Check sheet for the modelled part. Datum: model origin and axes. Units: mm. A direction names the side the tool comes from. Give positions to 0.01 mm unless a question says otherwise; leave off trailing zeros. Order: outer loops, then holes, each group sorted by start corner. A loop starts at its lowest first (then second) coordinate and runs counter-clockwise, first axis right, second up.
Item 1: Sectioned sample at D-D on z = 2.5. Count the separate pieces of the cut face and the enclosed holes in it, and give its area (3 significant figures).
Item 2: Release check for a two-part mould opening along X. For faces 5 (the flat face through (51.3, 6, 7)), 6 (the flat face through (5, 39.1, 5)), 7 (the flat face through (8.7, 18, 7)) record: released by +X, released by -X, zero draft, split by the parting line, or undercut.
Item 3: Sectioned sample at C-C on x = 4.5. Record the boundary of the cut face in (y, z).
Item 4: Access from +Z, -Z, +X, -X, +Y, -Y to the whole of each face (thin tool, end or side, straight path). Record for faces 1 (the flat face through (7, 26.4, 5)), 2 (the flat face through (47, 49.9, 7)), 3 (the flat face through (50, 25, 1)), 4 (the flat face through (47, 39.9, 7)).
Item 5: Gauge pin test, flat ends, axial feed: P1, Ø4.5, axis at x = 4, z = 9, coming from the +Y side; P2, Ø12, axis at x = 39, y = 31.5, coming from the +Z side; P3, Ø2, axis at x = 5, z = 6, coming from the -Y side. Record the tip position at first contact, or that the pin passes through.
Item 6: Material ranges on line 1 along Y through (x, z) = (4.5, 8.75); line 2 along Y through (x, z) = (2, 4.5); line 3 along X through (y, z) = (40, 7.75), recorded low to high.
Item 7: Sectioned sample at A-A on z = 10.5. Record the boundary of the cut face in (x, y).
Item 8: Sectioned sample at B-B on y = 4.5. Record the boundary of the cut face in (x, z), and give its area (3 significant figures).
from build123d import *

# Parameters (mm, degrees)
CROQUIS1_W              = 50
CROQUIS1_H              = 50
SALIENTE_EXTRUIR1_DEPTH = 1.2
CROQUIS2_W              = 9
CROQUIS2_H              = 10
SALIENTE_EXTRUIR2_DEPTH = 11.8
CROQUIS3_W              = 27.94
CROQUIS3_H              = 2.54
CROQUIS3_W_2            = 2.54
CROQUIS3_H_2            = 15.24
CROQUIS3_H_3            = 10.16
CROQUIS3_W_3            = 5.08
SALIENTE_EXTRUIR3_DEPTH = 8


with BuildPart() as part:
    # Croquis1 → Saliente-Extruir1 (new body)
    with BuildSketch(Plane.XY):
        with Locations((25, 25)):
            Rectangle(CROQUIS1_W, CROQUIS1_H)
    extrude(amount=SALIENTE_EXTRUIR1_DEPTH)

    # Croquis2 → Saliente-Extruir2 (add)
    with BuildSketch(Plane.XY.offset(1.2)):
        with Locations((46.8, 5.8)):
            Rectangle(CROQUIS2_W, CROQUIS2_H)
        with Locations((46.8, 18.4)):
            Rectangle(CROQUIS2_W, CROQUIS2_H)
        with Locations((46.8, 44.9)):
            Rectangle(CROQUIS2_W, CROQUIS2_H)
        with Locations((4.2, 44.9)):
            Rectangle(CROQUIS2_W, CROQUIS2_H)
        with Locations((4.2, 18.1)):
            Rectangle(CROQUIS2_W, CROQUIS2_H)
    extrude(amount=SALIENTE_EXTRUIR2_DEPTH)

    # Croquis3 → Saliente-Extruir3 (add)
    with BuildSketch(Plane.XY.offset(1.2)):
        with Locations((14.57, 2.07)):
            Rectangle(CROQUIS3_W, CROQUIS3_H)
        with Locations((4.57, 31.48)):
            Rectangle(CROQUIS3_W_2, CROQUIS3_H_2)
        with Locations((7.11, 31.48)):
            Rectangle(CROQUIS3_W_2, CROQUIS3_H_3)
        with Locations((46.66, 31.48)):
            Rectangle(CROQUIS3_W_3, CROQUIS3_H_3)
    extrude(amount=SALIENTE_EXTRUIR3_DEPTH)


solid = part.part
Report:
1. separate pieces: 8
1. enclosed holes: 0
1. area: 637 mm2
2. face 5: released by +X
2. face 6: zero draft
2. face 7: undercut
3. outline: (0, 0) - (50, 0) - (50, 1.2) - (49.9, 1.2) - (49.9, 13) - (39.9, 13) - (39.9, 1.2) - (39.1, 1.2) - (39.1, 9.2) - (23.86, 9.2) - (23.86, 1.2) - (23.1, 1.2) - (23.1, 13) - (13.1, 13) - (13.1, 1.2) - (3.34, 1.2) - (3.34, 9.2) - (0.8, 9.2) - (0.8, 1.2) - (0, 1.2) - close
4. face 1: +Z, +X
4. face 2: +Z, +X, -X, +Y
4. face 3: -Z, +X, +Y, -Y
4. face 4: +Z, +X, -X
5. P1: stops at y = 49.9
5. P2: stops at z = 9.2
5. P3: stops at y = 0.8
6. line 1: y = 0.8 to 3.34, 13.1 to 23.1, 23.86 to 39.1, 39.9 to 49.9
6. line 2: y = 0.8 to 3.34, 13.1 to 23.1, 39.9 to 49.9
6. line 3: x = -0.3 to 8.7, 42.3 to 51.3
7. outline: (-0.3, 13.1) - (8.7, 13.1) - (8.7, 23.1) - (-0.3, 23.1) - close; (-0.3, 39.9) - (8.7, 39.9) - (8.7, 49.9) - (-0.3, 49.9) - close; (42.3, 0.8) - (51.3, 0.8) - (51.3, 10.8) - (42.3, 10.8) - close; (42.3, 13.4) - (51.3, 13.4) - (51.3, 23.4) - (42.3, 23.4) - close; (42.3, 39.9) - (51.3, 39.9) - (51.3, 49.9) - (42.3, 49.9) - close
8. outline: (0, 0) - (50, 0) - (50, 1.2) - (51.3, 1.2) - (51.3, 13) - (42.3, 13) - (42.3, 1.2) - (0, 1.2) - close
8. area: 166 mm2
